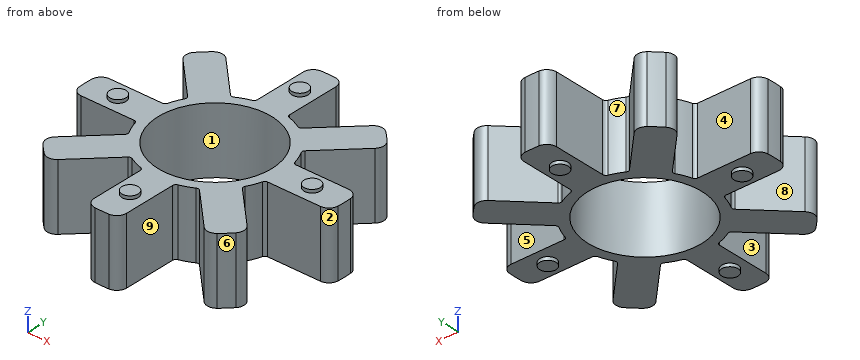
from build123d import *

# Parameters (mm, degrees)
SKETCH1_R           = 17.5
BOSS_EXTRUDE1_DEPTH = 10.25
SKETCH2_R           = 2.5
BOSS_EXTRUDE2_DEPTH = 1


with BuildPart() as part:
    # Sketch1 → Boss-Extrude1 (new body, symmetric)
    with BuildSketch(Plane.XY):
        with BuildLine():
            Line((-5, 36.945906404), (-5, 20.645822822))
            ThreePointArc((-5, 20.645822822), (-5.200290751, 20.04543535), (-5.720930233, 19.685551993))
            ThreePointArc((-5.720930233, 19.685551993), (-7.845010363, 18.939530416), (-9.874478744, 17.965095868))
            ThreePointArc((-9.874478744, 17.965095868), (-10.497102414, 17.851424122), (-11.063267415, 18.134335227))
            Line((-11.063267415, 18.134335227), (-22.589167049, 29.660234861))
            ThreePointArc((-22.589167049, 29.660234861), (-24.629376661, 30.537817825), (-26.714040425, 29.771799478))
            ThreePointArc((-26.714040425, 29.771799478), (-28.284271247, 28.284271247), (-29.771799478, 26.714040425))
            ThreePointArc((-29.771799478, 26.714040425), (-30.537817825, 24.629376661), (-29.660234861, 22.589167049))
            Line((-29.660234861, 22.589167049), (-18.134335227, 11.063267415))
            ThreePointArc((-18.134335227, 11.063267415), (-17.851424122, 10.497102414), (-17.965095868, 9.874478744))
            ThreePointArc((-17.965095868, 9.874478744), (-18.939530416, 7.845010363), (-19.685551993, 5.720930233))
            ThreePointArc((-19.685551993, 5.720930233), (-20.04543535, 5.200290751), (-20.645822822, 5))
            Line((-20.645822822, 5), (-36.945906404, 5))
            ThreePointArc((-36.945906404, 5), (-39.00909732, 4.177898814), (-39.941520437, 2.162162162))
            ThreePointArc((-39.941520437, 2.162162162), (-40, 0), (-39.941520437, -2.162162162))
            ThreePointArc((-39.941520437, -2.162162162), (-39.00909732, -4.177898814), (-36.945906404, -5))
            Line((-36.945906404, -5), (-20.645822822, -5))
            ThreePointArc((-20.645822822, -5), (-20.04543535, -5.200290751), (-19.685551993, -5.720930233))
            ThreePointArc((-19.685551993, -5.720930233), (-18.939530416, -7.845010363), (-17.965095868, -9.874478744))
            ThreePointArc((-17.965095868, -9.874478744), (-17.851424122, -10.497102414), (-18.134335227, -11.063267415))
            Line((-18.134335227, -11.063267415), (-29.660234861, -22.589167049))
            ThreePointArc((-29.660234861, -22.589167049), (-30.537817825, -24.629376661), (-29.771799478, -26.714040425))
            ThreePointArc((-29.771799478, -26.714040425), (-28.284271247, -28.284271247), (-26.714040425, -29.771799478))
            ThreePointArc((-26.714040425, -29.771799478), (-24.629376661, -30.537817825), (-22.589167049, -29.660234861))
            Line((-22.589167049, -29.660234861), (-11.063267415, -18.134335227))
            ThreePointArc((-11.063267415, -18.134335227), (-10.497102414, -17.851424122), (-9.874478744, -17.965095868))
            ThreePointArc((-9.874478744, -17.965095868), (-7.845010363, -18.939530416), (-5.720930233, -19.685551993))
            ThreePointArc((-5.720930233, -19.685551993), (-5.200290751, -20.04543535), (-5, -20.645822822))
            Line((-5, -20.645822822), (-5, -36.945906404))
            ThreePointArc((-5, -36.945906404), (-4.177898814, -39.00909732), (-2.162162162, -39.941520437))
            ThreePointArc((-2.162162162, -39.941520437), (0, -40), (2.162162162, -39.941520437))
            ThreePointArc((2.162162162, -39.941520437), (4.177898814, -39.00909732), (5, -36.945906404))
            Line((5, -36.945906404), (5, -20.645822822))
            ThreePointArc((5, -20.645822822), (5.200290751, -20.04543535), (5.720930233, -19.685551993))
            ThreePointArc((5.720930233, -19.685551993), (7.845010363, -18.939530416), (9.874478744, -17.965095868))
            ThreePointArc((9.874478744, -17.965095868), (10.497102414, -17.851424122), (11.063267415, -18.134335227))
            Line((11.063267415, -18.134335227), (22.589167049, -29.660234861))
            ThreePointArc((22.589167049, -29.660234861), (24.629376661, -30.537817825), (26.714040425, -29.771799478))
            ThreePointArc((26.714040425, -29.771799478), (28.284271247, -28.284271247), (29.771799478, -26.714040425))
            ThreePointArc((29.771799478, -26.714040425), (30.537817825, -24.629376661), (29.660234861, -22.589167049))
            Line((29.660234861, -22.589167049), (18.134335227, -11.063267415))
            ThreePointArc((18.134335227, -11.063267415), (17.851424122, -10.497102414), (17.965095868, -9.874478744))
            ThreePointArc((17.965095868, -9.874478744), (18.939530416, -7.845010363), (19.685551993, -5.720930233))
            ThreePointArc((19.685551993, -5.720930233), (20.04543535, -5.200290751), (20.645822822, -5))
            Line((20.645822822, -5), (36.945906404, -5))
            ThreePointArc((36.945906404, -5), (39.00909732, -4.177898814), (39.941520437, -2.162162162))
            ThreePointArc((39.941520437, -2.162162162), (40, 0), (39.941520437, 2.162162162))
            ThreePointArc((39.941520437, 2.162162162), (39.00909732, 4.177898814), (36.945906404, 5))
            Line((36.945906404, 5), (20.645822822, 5))
            ThreePointArc((20.645822822, 5), (20.04543535, 5.200290751), (19.685551993, 5.720930233))
            ThreePointArc((19.685551993, 5.720930233), (18.939530416, 7.845010363), (17.965095868, 9.874478744))
            ThreePointArc((17.965095868, 9.874478744), (17.851424122, 10.497102414), (18.134335227, 11.063267415))
            Line((18.134335227, 11.063267415), (29.660234861, 22.589167049))
            ThreePointArc((29.660234861, 22.589167049), (30.537817825, 24.629376661), (29.771799478, 26.714040425))
            ThreePointArc((29.771799478, 26.714040425), (28.284271247, 28.284271247), (26.714040425, 29.771799478))
            ThreePointArc((26.714040425, 29.771799478), (24.629376661, 30.537817825), (22.589167049, 29.660234861))
            Line((22.589167049, 29.660234861), (11.063267415, 18.134335227))
            ThreePointArc((11.063267415, 18.134335227), (10.497102414, 17.851424122), (9.874478744, 17.965095868))
            ThreePointArc((9.874478744, 17.965095868), (7.845010363, 18.939530416), (5.720930233, 19.685551993))
            ThreePointArc((5.720930233, 19.685551993), (5.200290751, 20.04543535), (5, 20.645822822))
            Line((5, 20.645822822), (5, 36.945906404))
            ThreePointArc((5, 36.945906404), (4.177898814, 39.00909732), (2.162162162, 39.941520437))
            ThreePointArc((2.162162162, 39.941520437), (0, 40), (-2.162162162, 39.941520437))
            ThreePointArc((-2.162162162, 39.941520437), (-4.177898814, 39.00909732), (-5, 36.945906404))
        make_face()
        Circle(SKETCH1_R, mode=Mode.SUBTRACT)
    extrude(amount=BOSS_EXTRUDE1_DEPTH, both=True)

    # Sketch2 → Boss-Extrude2 (add)
    with BuildSketch(Plane.XY.offset(10.25)):
        with Locations((0, 30)):
            Circle(SKETCH2_R)
        with Locations((30, 0)):
            Circle(SKETCH2_R)
        with Locations((0, -30)):
            Circle(SKETCH2_R)
        with Locations((-30, 0)):
            Circle(SKETCH2_R)
    boss_extrude2 = extrude(amount=BOSS_EXTRUDE2_DEPTH)

    # Mirror1: Boss-Extrude2 across plane
    add(boss_extrude2.mirror(Plane.XY))


solid = part.part
Build history of the part. All positions in model axes, mm. Face numbers are marked on the shaded views. A direction names the side the tool comes from. Round coordinates to 2 decimals unless told otherwise and drop trailing zeros. Loops run counter-clockwise (first coordinate to the right, second up) from the corner with the lowest first, then second, coordinate; pieces in that order, holes last. Notation, with made-up numbers: (-8, 37.25) -> (31, 37.25) arc R9 cw to (31, 49.25) -> close; hole circle Ø1 at (16.5, 61). An arc over 180 degrees is marked (long way). One line per item, written item: value. Start each with the question number.
Q1. Cut at A-A on y = 0. List the corners of the cut face in (x, z), plus the area to 4 significant figures.
Q2. Cut at C-C on y = -28.5. List the corners of the cut face in (x, z), plus the area to 3 significant figures.
Q3. Probe line 1 along Y through (x, z) = (24.5, 4.25); line 2 along X through (y, z) = (-22, 1.25); line 3 along Y through (x, z) = (27, 7.25). List the from-to ranges inside material, lowest first.
Q4. Two-plate mould, pull along X, no slides. Class the marked faces 1, 2, 3 and 4: released by +X, released by -X, zero draft, split by the parting line, or undercut.
Q5. Cut at B-B on x = -1. List the corners of the cut face in (y, z), plus the area to 3 significant figures.
Q6. 3-axis set-ups, long thin cutter, end or side, ignore diameter. For the marked faces 5, 6, 7, 8 and 9: which of +Z, -Z, +X, -X, +Y, -Y reach the whole face in a straight line?
Q7. Cut at D-D on x = -15. List the corners of the cut face in (y, z), plus the area to 3 significant figures.
Q8. Drop flat-ended pins along their axis: pin 1 Ø1.5 at (x, z) = (14, -8) entering from +Y; pin 2 Ø8 at (y, z) = (-25, 3) entering from +X; pin 3 Ø5 at (x, z) = (-25.5, 3.5) entering from -Y; pin 4 Ø24 at (x, y) = (-2.5, -3.5) entering from -Z. Give the stop position or say it passes through.
Computed:
1. outline: (-40, -10.25) -> (-32.5, -10.25) -> (-32.5, -11.25) -> (-27.5, -11.25) -> (-27.5, -10.25) -> (-17.5, -10.25) -> (-17.5, 10.25) -> (-27.5, 10.25) -> (-27.5, 11.25) -> (-32.5, 11.25) -> (-32.5, 10.25) -> (-40, 10.25) -> close; (17.5, -10.25) -> (27.5, -10.25) -> (27.5, -11.25) -> (32.5, -11.25) -> (32.5, -10.25) -> (40, -10.25) -> (40, 10.25) -> (32.5, 10.25) -> (32.5, 11.25) -> (27.5, 11.25) -> (27.5, 10.25) -> (17.5, 10.25) -> close
1. area: 942.5 mm²
2. outline: (-28.07, -10.25) -> (-21.43, -10.25) -> (-21.43, 10.25) -> (-28.07, 10.25) -> close; (-5, -10.25) -> (-2, -10.25) -> (-2, -11.25) -> (2, -11.25) -> (2, -10.25) -> (5, -10.25) -> (5, 10.25) -> (2, 10.25) -> (2, 11.25) -> (-2, 11.25) -> (-2, 10.25) -> (-5, 10.25) -> close; (21.43, -10.25) -> (28.07, -10.25) -> (28.07, 10.25) -> (21.43, 10.25) -> close
2. area: 485 mm²
3. line 1: -30.53 to -17.43, -5 to 5, 17.43 to 30.53
3. line 2: -29.07 to -14.93, -5 to 5, 14.93 to 29.07
3. line 3: -29.51 to -19.93, -5 to 5, 19.93 to 29.51
4. face 1: undercut
4. face 2: released by +X
4. face 3: undercut
4. face 4: zero draft
5. outline: (-39.99, -10.25) -> (-32.29, -10.25) -> (-32.29, -11.25) -> (-27.71, -11.25) -> (-27.71, -10.25) -> (-17.47, -10.25) -> (-17.47, 10.25) -> (-27.71, 10.25) -> (-27.71, 11.25) -> (-32.29, 11.25) -> (-32.29, 10.25) -> (-39.99, 10.25) -> close; (17.47, -10.25) -> (27.71, -10.25) -> (27.71, -11.25) -> (32.29, -11.25) -> (32.29, -10.25) -> (39.99, -10.25) -> (39.99, 10.25) -> (32.29, 10.25) -> (32.29, 11.25) -> (27.71, 11.25) -> (27.71, 10.25) -> (17.47, 10.25) -> close
5. area: 941 mm²
6. face 5: +Z, -Z, +X
6. face 6: +Z, -Z, +X, -Y
6. face 7: +Z, -Z, +Y
6. face 8: +Z, -Z, -X
6. face 9: +Z, -Z, -Y
7. outline: (-22.07, -10.25) -> (-9.01, -10.25) -> (-9.01, 10.25) -> (-22.07, 10.25) -> close; (9.01, -10.25) -> (22.07, -10.25) -> (22.07, 10.25) -> (9.01, 10.25) -> close
7. area: 535 mm²
8. pin 1: y = 21.82
8. pin 2: x = 30.54
8. pin 3: y = -30.54
8. pin 4: through
